Work out the finished part from the listing and answer in its coordinate system (mm). A direction names the side the tool comes from. Coordinates: 2 decimals unless noted, no trailing zeros. Loops run counter-clockwise (first coordinate to the right, second up) from the corner with the lowest first, then second, coordinate; pieces in that order, holes last. Notation, with made-up numbers: (83.5, -12.75) -> (92.5, -12.75) arc R13 cw to (92.5, 7.25) -> close; hole circle Ø11 at (89, 43). An arc over 180 degrees is marked (long way). One line per question, with ' | ' between items.
```python
from build123d import *

# Parameters (mm, degrees)
SKETCH2_W           = 44.704
SKETCH2_H           = 35.052
BOSS_EXTRUDE1_DEPTH = 119.126
SKETCH4_W           = 51.054
SKETCH4_H           = 41.402
SKETCH4_W_2         = 47.752
SKETCH4_H_2         = 38.354
BOSS_EXTRUDE2_DEPTH = 115.951
SKETCH5_W           = 51.054
SKETCH5_H           = 41.402
BOSS_EXTRUDE3_DEPTH = 3.175
CUT_EXTRUDE1_DEPTH  = 6.35
CUT_EXTRUDE2_DEPTH  = 132.811951465
CUT_EXTRUDE3_DEPTH  = 130.93059219


with BuildPart() as part:
    # Sketch2 → Boss-Extrude1 (new body)
    with BuildSketch(Plane.XY):
        Polygon((-29.730268616, 22.430738007), (18.021731384, 22.430738007), (18.021731384, -15.923261993), (-29.730268616, -15.923261993), (-29.730268616, -15.068411042), align=None)
        with Locations((-5.790768616, 3.317238007)):
            Rectangle(SKETCH2_W, SKETCH2_H, mode=Mode.SUBTRACT)
    extrude(amount=BOSS_EXTRUDE1_DEPTH)

    # Sketch4 → Boss-Extrude2 (add)
    with BuildSketch(Plane(origin=(0, 0, 0), x_dir=(-1, 0, 0), z_dir=(0, 0, -1))):
        with Locations((5.727268616, 3.317238007)):
            Rectangle(SKETCH4_W, SKETCH4_H)
        with Locations((5.854268616, 3.253738007)):
            Rectangle(SKETCH4_W_2, SKETCH4_H_2, mode=Mode.SUBTRACT)
    extrude(amount=-BOSS_EXTRUDE2_DEPTH)

    # Sketch5 → Boss-Extrude3 (add)
    with BuildSketch(Plane(origin=(0, 0, 0), x_dir=(-1, 0, 0), z_dir=(0, 0, -1))):
        with Locations((5.727268616, 3.317238007)):
            Rectangle(SKETCH5_W, SKETCH5_H)
    extrude(amount=-BOSS_EXTRUDE3_DEPTH)

    # Sketch6 → Cut-Extrude1 (cut)
    with BuildSketch(Plane.XY.offset(3.175)):
        with BuildLine():
            Line((-21.094268616, 17.668238007), (9.639731384, 17.668238007))
            ThreePointArc((9.639731384, 17.668238007), (12.33380822, 16.552314843), (13.449731384, 13.858238007))
            Line((13.449731384, 13.858238007), (13.449731384, -7.223761993))
            ThreePointArc((13.449731384, -7.223761993), (12.33380822, -9.91783883), (9.639731384, -11.033761993))
            Line((9.639731384, -11.033761993), (-21.094268616, -11.033761993))
            ThreePointArc((-21.094268616, -11.033761993), (-23.788345453, -9.91783883), (-24.904268616, -7.223761993))
            Line((-24.904268616, -7.223761993), (-24.904268616, 13.858238007))
            ThreePointArc((-24.904268616, 13.858238007), (-23.788345453, 16.552314843), (-21.094268616, 17.668238007))
        make_face()
    extrude(amount=-CUT_EXTRUDE1_DEPTH, mode=Mode.SUBTRACT)

    # Sketch7 → Cut-Extrude2 (cut, through all)
    with BuildSketch(Plane.ZY.offset(-19.799731384)):
        with BuildLine():
            Line((23.847961018, -11.033761993), (90.515538982, -11.033761993))
            ThreePointArc((90.515538982, -11.033761993), (94.889610614, -10.16370505), (98.597769491, -7.685992502))
            Line((98.597769491, -7.685992502), (106.906923164, 0.62316117))
            ThreePointArc((106.906923164, 0.62316117), (108.022846327, 3.317238007), (106.906923164, 6.011314843))
            Line((106.906923164, 6.011314843), (98.597769491, 14.320468515))
            ThreePointArc((98.597769491, 14.320468515), (94.889610614, 16.798181063), (90.515538982, 17.668238007))
            Line((90.515538982, 17.668238007), (23.847961018, 17.668238007))
            ThreePointArc((23.847961018, 17.668238007), (19.473889386, 16.798181063), (15.765730509, 14.320468515))
            Line((15.765730509, 14.320468515), (7.456576836, 6.011314843))
            ThreePointArc((7.456576836, 6.011314843), (6.340653673, 3.317238007), (7.456576836, 0.62316117))
            Line((7.456576836, 0.62316117), (15.765730509, -7.685992502))
            ThreePointArc((15.765730509, -7.685992502), (19.473889386, -10.16370505), (23.847961018, -11.033761993))
        make_face()
    extrude(amount=CUT_EXTRUDE2_DEPTH, mode=Mode.SUBTRACT)

    # Sketch8 → Cut-Extrude3 (cut, through all)
    with BuildSketch(Plane(origin=(0, 24.018238007, 0), x_dir=(1, 0, 0), z_dir=(0, 1, 0))):
        with BuildLine():
            Line((9.729987505, -20.219756121), (-1.237140556, -9.252628061))
            ThreePointArc((-1.237140556, -9.252628061), (-5.727268616, -7.392756121), (-10.217396677, -9.252628061))
            Line((-10.217396677, -9.252628061), (-21.184524737, -20.219756121))
            ThreePointArc((-21.184524737, -20.219756121), (-23.937538679, -24.339932651), (-24.904268616, -29.200012242))
            Line((-24.904268616, -29.200012242), (-24.904268616, -85.163487758))
            ThreePointArc((-24.904268616, -85.163487758), (-23.937538679, -90.023567349), (-21.184524737, -94.143743879))
            Line((-21.184524737, -94.143743879), (-10.217396677, -105.110871939))
            ThreePointArc((-10.217396677, -105.110871939), (-5.727268616, -106.970743879), (-1.237140556, -105.110871939))
            Line((-1.237140556, -105.110871939), (9.729987505, -94.143743879))
            ThreePointArc((9.729987505, -94.143743879), (12.483001447, -90.023567349), (13.449731384, -85.163487758))
            Line((13.449731384, -85.163487758), (13.449731384, -29.200012242))
            ThreePointArc((13.449731384, -29.200012242), (12.483001447, -24.339932651), (9.729987505, -20.219756121))
        make_face()
    extrude(amount=-CUT_EXTRUDE3_DEPTH, mode=Mode.SUBTRACT)


solid = part.part
```
1) Find section B-B (x = -3.5). Write down the section's boundary in (y, z) (3 decimals).
Check values:
outline: (-17.384, 0) -> (-11.034, 0) -> (-11.034, 3.175) -> (-14.209, 3.175) -> (-14.209, 7.796) -> (-17.384, 7.796) -> close; (-17.384, 106.567) -> (-14.209, 106.567) -> (-14.209, 119.126) -> (-15.923, 119.126) -> (-15.923, 115.951) -> (-17.384, 115.951) -> close; (17.668, 0) -> (24.018, 0) -> (24.018, 7.796) -> (20.843, 7.796) -> (20.843, 3.175) -> (17.668, 3.175) -> close; (20.843, 106.567) -> (24.018, 106.567) -> (24.018, 115.951) -> (22.431, 115.951) -> (22.431, 119.126) -> (20.843, 119.126) -> close
2) Flat-ended cylindrical pins translate along their axes: pin 1 (3 mm diameter, centred on x = 11.5, y = 11.5, fed in from -Z); pin 2 (1.6 mm diameter, centred on x = 3, z = 117.5, fed in from +Y); pin 3 (5 mm diameter, centred on x = 5, y = -10, fed in from +Z) (3 decimals); pin 4 (3.5 mm diameter, centred on x = -11.5, z = 118.5, fed in from -Y). Find the tip coordinate at first contact, or state that the pin passes through.
Check values:
pin 1: passes through | pin 2: stops at y = 22.43 | pin 3: stops at z = 3.175 | pin 4: stops at y = -15.92
3) For faces 1 (the face through (12.36, -9.89, 1.61)), 2 (the face through (18, 17, 20)), 3 (the face through (-28, 24.018, 57)), 4 (the face through (14, -14.209, 60)), 5 (the face through (12.456, -15.774, 90.088)), determine the directions among +Z, -Z, +X, -X, +Y, -Y from which every point of the face is accessible in a straight line to the end or side of a thin tool.
Check values:
face 1: +Z, -Z | face 2: +X, -X | face 3: +Z, -Z, +X, -X, +Y | face 4: +Z | face 5: +Y, -Y
4) Find section C-C (x = -27). Write down the section's boundary in (y, z) (3 decimals), plus the area to 3 significant figures.
Check values:
outline: (-17.384, 0) -> (24.018, 0) -> (24.018, 115.951) -> (22.431, 115.951) -> (22.431, 119.126) -> (20.843, 119.126) -> (20.843, 3.175) -> (-14.209, 3.175) -> (-14.209, 119.126) -> (-15.923, 119.126) -> (-15.923, 115.951) -> (-17.384, 115.951) -> close | area: 858 mm^2
5) Find the intervals of material crossed by line 1 along X through (y, z) = (19, 48.5); line 2 along Y through (x, z) = (-25.5, 22.5); line 3 along Z through (x, y) = (-29, 12), in increasing order.
Check values:
line 1: x = -31.25 to -28.14, 16.56 to 19.8 | line 2: y = -17.38 to -14.21, 20.84 to 24.02 | line 3: z = 0 to 13.45, 100.92 to 119.13
6) The mould has two halves that part along Z. Classify faces 6 (the face through (-5, -12, 3.175)), 7 (the face through (18.022, 4, 118)), 8 (the face through (-5.8, 22.45, 106.97)): released by +Z, released by -Z, zero draft, split by the parting line, or undercut.
Check values:
face 6: released by +Z | face 7: zero draft | face 8: undercut
7) Find section A-A (z = 36). Write down the section's boundary in (x, y).
Check values:
outline: (-31.25, -17.38) -> (-24.9, -17.38) -> (-24.9, -14.21) -> (-28.14, -14.21) -> (-28.14, -11.03) -> (-31.25, -11.03) -> close; (-31.25, 17.67) -> (-28.14, 17.67) -> (-28.14, 20.84) -> (-24.9, 20.84) -> (-24.9, 24.02) -> (-31.25, 24.02) -> close; (13.45, -17.38) -> (19.8, -17.38) -> (19.8, -11.03) -> (16.56, -11.03) -> (16.56, -14.21) -> (13.45, -14.21) -> close; (13.45, 20.84) -> (16.56, 20.84) -> (16.56, 17.67) -> (19.8, 17.67) -> (19.8, 24.02) -> (13.45, 24.02) -> close
